Could you check a few things on this model? Use its own coordinates, in mm. Face numbers are marked on the shaded views. A direction names the side the tool comes from. Round coordinates to 2 decimals unless told otherwise and drop trailing zeros. Write each loop counter-clockwise with the first axis right and the second up, starting at its lowest first coordinate (ties: lowest second). Pieces come first, ordered by that corner, then holes. Notation, with made-up numbers: (-16.75, -39.75) - (35.25, -39.75) arc R22 ccw to (35.25, -26.75) - close; hole circle Ø2 at (61, 89.25). An arc over 180 degrees is marked (long way). Put each result on its own line as item: value.
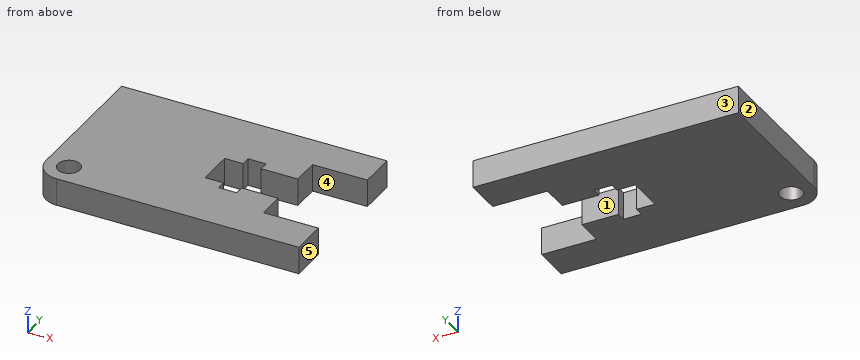
from build123d import *

# Parameters (mm, degrees)
F0_R     = 3.07505
F1_DEPTH = 7.62


with BuildPart() as f1:
    # F0 (on Top) → F1 (new body)
    with BuildSketch(Plane.XY):
        with BuildLine():
            Line((73.66, 0), (0, 0))
            Line((0, 0), (0, -39.215128))
            ThreePointArc((0, -39.215128), (1.85471, -43.700088), (6.335392, -45.565111))
            Line((6.335392, -45.565111), (73.664084, -45.72))
            Line((73.664084, -45.72), (73.664084, -35.56))
            Line((73.664084, -35.56), (58.417156, -35.56))
            Line((58.417156, -35.56), (58.417156, -27.94))
            Line((58.417156, -27.94), (48.26, -27.94))
            Line((48.26, -27.94), (48.26, -30.48))
            Line((48.26, -30.48), (43.18, -30.48))
            Line((43.18, -30.48), (43.18, -27.94))
            Line((43.18, -27.94), (38.1, -27.94))
            Line((38.1, -27.94), (38.1, -17.78))
            Line((38.1, -17.78), (43.18, -17.78))
            Line((43.18, -17.78), (43.18, -15.24))
            Line((43.18, -15.24), (48.26, -15.24))
            Line((48.26, -15.24), (48.26, -17.78))
            Line((48.26, -17.78), (58.42, -17.78))
            Line((58.42, -17.78), (58.42, -10.16))
            Line((58.42, -10.16), (73.66, -10.16))
            Line((73.66, -10.16), (73.66, 0))
        make_face()
        with Locations((6.35, -39.215128)):
            Circle(F0_R, mode=Mode.SUBTRACT)
    extrude(amount=F1_DEPTH)


solid = f1.part
(1) Imagine slicing it at A-A, the plane x = 66. List the corners of the cut face in (y, z) for me.
Values found:
outline: (-45.7, 0) - (-35.56, 0) - (-35.56, 7.62) - (-45.7, 7.62) - close; (-10.16, 0) - (0, 0) - (0, 7.62) - (-10.16, 7.62) - close
(2) I'm going to push flat-ended pins straight in: pin 1 (5.5 mm diameter, centred on x = 6.35, y = -39.22, fed in from -Z); pin 2 (2.5 mm diameter, centred on y = -15, z = 3, fed in from +X). Where does each tip first touch, or does it pass through?
Values found:
pin 1: passes through
pin 2: stops at x = 58.42
(3) Imagine slicing it at C-C, the plane y = -40. List the corners of the cut face in (x, z) for me, then the cut area to 3 significant figures.
Values found:
outline: (0.05, 0) - (3.38, 0) - (3.38, 7.62) - (0.05, 7.62) - close; (9.32, 0) - (73.66, 0) - (73.66, 7.62) - (9.32, 7.62) - close
area: 516 mm^2
(4) If we mould it in two halves opening along Y, with no side actions, what happens to the marked faces 1, 2 and 3? For each: pulls with the +Y half, pulls with the -Y half, needs draft (parallel to the pull), parting line crosses it, or undercut.
Values found:
face 1: undercut
face 2: needs draft
face 3: pulls with the +Y half
(5) For the marked faces 4 and 5, which set-ups out of +Z, -Z, +X, -X, +Y, -Y let a thin tool reach every point of the face, with its end or its side?
Values found:
face 4: +Z, -Z, +X
face 5: +Z, -Z, +X, +Y, -Y
(6) Imagine slicing it at B-B, the plane z = 1. List the corners of the cut face in (x, y) for me.
Values found:
outline: (0, -39.22) arc R6.35 ccw to (6.34, -45.57) - (73.66, -45.72) - (73.66, -35.56) - (58.42, -35.56) - (58.42, -27.94) - (48.26, -27.94) - (48.26, -30.48) - (43.18, -30.48) - (43.18, -27.94) - (38.1, -27.94) - (38.1, -17.78) - (43.18, -17.78) - (43.18, -15.24) - (48.26, -15.24) - (48.26, -17.78) - (58.42, -17.78) - (58.42, -10.16) - (73.66, -10.16) - (73.66, 0) - (0, 0) - close; hole circle Ø6.15 at (6.35, -39.22)
(7) Please list where these lines run through material, in increasing order: probe 1 along Y at (x, z) = (6.35, 2); probe 2 along X at (y, z) = (-6.5, 3.5); probe 3 along X at (y, z) = (-15, 5). Write a range as from..to.
Values found:
probe 1: y = -45.57..-42.29, -36.14..0
probe 2: x = 0..73.66
probe 3: x = 0..58.42
(8) Imagine slicing it at D-D, the plane y = -12.5. List the corners of the cut face in (x, z) for me.
Values found:
outline: (0, 0) - (58.42, 0) - (58.42, 7.62) - (0, 7.62) - close
